Check sheet for the modelled part. Datum: model origin and axes. Units: mm. Face numbers are marked on the shaded views. A direction names the side the tool comes from. Give positions to 0.01 mm unless a question says otherwise; leave off trailing zeros. Write each loop counter-clockwise with the first axis right and the second up, starting at its lowest first coordinate (ties: lowest second). Pieces come first, ordered by that corner, then holes.
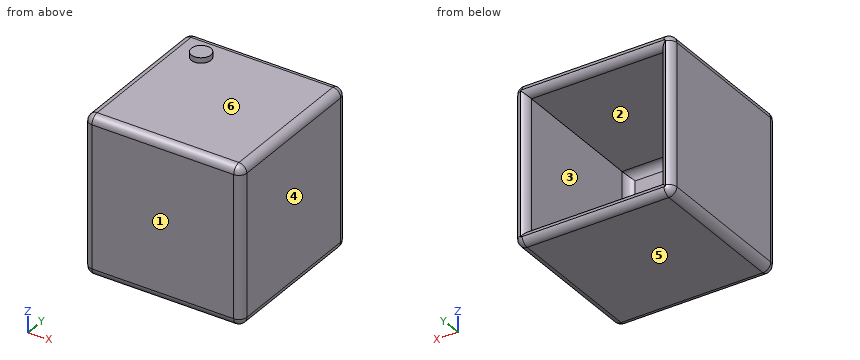
from build123d import *

# Parameters (mm, degrees)
F0_W         = 100
F0_H         = 100
F1_DEPTH     = 100
F2_R         = 5
F3_W         = 84.485553205
F3_H         = 83.5751444101
F4_DEPTH     = 96.9
F5_R         = 5
F6_T1_DEPTH  = 84.485553205
F6_T3_DEPTH  = 83.5751444101
F6_T9_DEPTH  = 96.985553205
F6_T13_DEPTH = 96.0751444101
F6_T20_DEPTH = 96.985553205
F6_T24_DEPTH = 96.0751444101
F6_T31_DEPTH = 96.0751444101
F6_T35_DEPTH = 96.985553205
F6_T42_DEPTH = 96.0751444101
F6_T46_DEPTH = 96.985553205
F7_R         = 6.1934205271
F8_DEPTH     = 3.4


# Not quite as in the source:
# - a fillet or chamfer that OpenCascade refuses, or shapes differently, is made with other operations: its cross-section is extruded or revolved along the edge and cut away or added


with BuildPart() as f1:
    # F0 (on Front) → F1 (new body)
    with BuildSketch(Plane.XZ):
        Rectangle(F0_W, F0_H)
    extrude(amount=F1_DEPTH)

    # F2
    f2_edges = [f1.edges().sort_by_distance(p)[0] for p in [
        (0, -100, 50),
        (-50, -100, 0),
        (0, -100, -50),
        (50, -100, 0),
        (50, -50, -50),
        (-50, -50, -50),
        (0, 0, -50),
        (50, -50, 50),
        (-50, -50, 50),
        (0, 0, 50),
        (50, 0, 0),
        (-50, 0, 0),
    ]]
    fillet(f2_edges, radius=F2_R)

    # F3 (on Front) → F4 (cut)
    with BuildSketch(Plane.XZ):
        Rectangle(F3_W, F3_H)
    extrude(amount=F4_DEPTH, mode=Mode.SUBTRACT)

    # F5
    f5_edges = [f1.edges().sort_by_distance(p)[0] for p in [
        (0, -96.9, -41.787572),
        (42.242777, -96.9, 0),
        (0, -96.9, 41.787572),
        (-42.242777, -96.9, 0),
    ]]
    fillet(f5_edges, radius=F5_R)

    # F6: fillet of radius 5 on 8 edges, made by hand

    # F6_s2 → F6_t1 (cut)
    with BuildSketch(Plane.YZ.offset(-42.2427766025)):
        with BuildLine():
            ThreePointArc((-5, -41.7875722051), (-1.4644660941, -43.2520382991), (0, -46.7875722051))
            Line((0, -46.7875722051), (0, -41.7875722051))
            Line((0, -41.7875722051), (-5, -41.7875722051))
        make_face()
        with BuildLine():
            ThreePointArc((0, 46.7875722051), (-1.4644660941, 43.2520382991), (-5, 41.7875722051))
            Line((-5, 41.7875722051), (0, 41.7875722051))
            Line((0, 41.7875722051), (0, 46.7875722051))
        make_face()
    extrude(amount=F6_T1_DEPTH, mode=Mode.SUBTRACT)

    # F6_s4 → F6_t3 (cut)
    with BuildSketch(Plane.XY.offset(-41.7875722051)):
        with BuildLine():
            ThreePointArc((47.2427766025, 0), (43.7072426966, -1.4644660941), (42.2427766025, -5))
            Line((42.2427766025, -5), (42.2427766025, 0))
            Line((42.2427766025, 0), (47.2427766025, 0))
        make_face()
        with BuildLine():
            ThreePointArc((-42.2427766025, -5), (-43.7072426966, -1.4644660941), (-47.2427766025, 0))
            Line((-47.2427766025, 0), (-42.2427766025, 0))
            Line((-42.2427766025, 0), (-42.2427766025, -5))
        make_face()
    extrude(amount=F6_T3_DEPTH, mode=Mode.SUBTRACT)


with BuildPart() as f6_tool7:
    # F6_s8 → F6_t9 (new body)
    with BuildSketch(Plane.YZ.offset(-54.7427766025)):
        with BuildLine():
            ThreePointArc((-5, -41.7875722051), (-1.4644660941, -43.2520382991), (0, -46.7875722051))
            Line((0, -46.7875722051), (0, -41.7875722051))
            Line((0, -41.7875722051), (-5, -41.7875722051))
        make_face()
    extrude(amount=F6_T9_DEPTH)

    split(bisect_by=Plane.YZ.offset(-42.2427766025), keep=Keep.BOTTOM)


with BuildPart() as f6_tool11:
    # F6_s12 → F6_t13 (new body)
    with BuildSketch(Plane.XY.offset(41.7875722051)):
        with BuildLine():
            ThreePointArc((-42.2427766025, -5), (-43.7072426966, -1.4644660941), (-47.2427766025, 0))
            Line((-47.2427766025, 0), (-42.2427766025, 0))
            Line((-42.2427766025, 0), (-42.2427766025, -5))
        make_face()
    extrude(amount=-F6_T13_DEPTH)

    split(bisect_by=Plane.XY.offset(-41.7875722051), keep=Keep.BOTTOM)


with BuildPart() as f6_tool7_1:
    add(f6_tool7.part)

    # F6_t15: intersect F6_tool11
    add(f6_tool11.part, mode=Mode.INTERSECT)


with BuildPart() as f1_1:
    add(f1.part)

    # F6_t5: cut F6_tool7
    add(f6_tool7_1.part, mode=Mode.SUBTRACT)


with BuildPart() as f6_tool18:
    # F6_s19 → F6_t20 (new body)
    with BuildSketch(Plane.YZ.offset(-42.2427766025)):
        with BuildLine():
            ThreePointArc((-5, -41.7875722051), (-1.4644660941, -43.2520382991), (0, -46.7875722051))
            Line((0, -46.7875722051), (0, -41.7875722051))
            Line((0, -41.7875722051), (-5, -41.7875722051))
        make_face()
    extrude(amount=F6_T20_DEPTH)

    split(bisect_by=Plane.YZ.offset(42.2427766025), keep=Keep.TOP)


with BuildPart() as f6_tool22:
    # F6_s23 → F6_t24 (new body)
    with BuildSketch(Plane.XY.offset(-54.2875722051)):
        with BuildLine():
            ThreePointArc((47.2427766025, 0), (43.7072426966, -1.4644660941), (42.2427766025, -5))
            Line((42.2427766025, -5), (42.2427766025, 0))
            Line((42.2427766025, 0), (47.2427766025, 0))
        make_face()
    extrude(amount=F6_T24_DEPTH)

    split(bisect_by=Plane.XY.offset(-41.7875722051), keep=Keep.BOTTOM)


with BuildPart() as f6_tool18_1:
    add(f6_tool18.part)

    # F6_t26: intersect F6_tool22
    add(f6_tool22.part, mode=Mode.INTERSECT)


with BuildPart() as f1_2:
    add(f1_1.part)

    # F6_t16: cut F6_tool18
    add(f6_tool18_1.part, mode=Mode.SUBTRACT)


with BuildPart() as f6_tool29:
    # F6_s30 → F6_t31 (new body)
    with BuildSketch(Plane.XY.offset(-41.7875722051)):
        with BuildLine():
            ThreePointArc((47.2427766025, 0), (43.7072426966, -1.4644660941), (42.2427766025, -5))
            Line((42.2427766025, -5), (42.2427766025, 0))
            Line((42.2427766025, 0), (47.2427766025, 0))
        make_face()
    extrude(amount=F6_T31_DEPTH)

    split(bisect_by=Plane.XY.offset(41.7875722051), keep=Keep.TOP)


with BuildPart() as f6_tool33:
    # F6_s34 → F6_t35 (new body)
    with BuildSketch(Plane.YZ.offset(54.7427766025)):
        with BuildLine():
            ThreePointArc((0, 46.7875722051), (-1.4644660941, 43.2520382991), (-5, 41.7875722051))
            Line((-5, 41.7875722051), (0, 41.7875722051))
            Line((0, 41.7875722051), (0, 46.7875722051))
        make_face()
    extrude(amount=-F6_T35_DEPTH)

    split(bisect_by=Plane.YZ.offset(42.2427766025), keep=Keep.TOP)


with BuildPart() as f6_tool29_1:
    add(f6_tool29.part)

    # F6_t37: intersect F6_tool33
    add(f6_tool33.part, mode=Mode.INTERSECT)


with BuildPart() as f1_3:
    add(f1_2.part)

    # F6_t27: cut F6_tool29
    add(f6_tool29_1.part, mode=Mode.SUBTRACT)


with BuildPart() as f6_tool40:
    # F6_s41 → F6_t42 (new body)
    with BuildSketch(Plane.XY.offset(54.2875722051)):
        with BuildLine():
            ThreePointArc((-42.2427766025, -5), (-43.7072426966, -1.4644660941), (-47.2427766025, 0))
            Line((-47.2427766025, 0), (-42.2427766025, 0))
            Line((-42.2427766025, 0), (-42.2427766025, -5))
        make_face()
    extrude(amount=-F6_T42_DEPTH)

    split(bisect_by=Plane.XY.offset(41.7875722051), keep=Keep.TOP)


with BuildPart() as f6_tool44:
    # F6_s45 → F6_t46 (new body)
    with BuildSketch(Plane.YZ.offset(42.2427766025)):
        with BuildLine():
            ThreePointArc((0, 46.7875722051), (-1.4644660941, 43.2520382991), (-5, 41.7875722051))
            Line((-5, 41.7875722051), (0, 41.7875722051))
            Line((0, 41.7875722051), (0, 46.7875722051))
        make_face()
    extrude(amount=-F6_T46_DEPTH)

    split(bisect_by=Plane.YZ.offset(-42.2427766025), keep=Keep.BOTTOM)


with BuildPart() as f6_tool40_1:
    add(f6_tool40.part)

    # F6_t48: intersect F6_tool44
    add(f6_tool44.part, mode=Mode.INTERSECT)


with BuildPart() as f1_4:
    add(f1_3.part)

    # F6_t38: cut F6_tool40
    add(f6_tool40_1.part, mode=Mode.SUBTRACT)

    # F7 (on face) → F8 (join)
    with BuildSketch(Plane.XY.offset(50)):
        with Locations((-29.7398809344, -18.3617770672)):
            Circle(F7_R)
    extrude(amount=F8_DEPTH)


solid = f1_4.part
1) Access from +Z, -Z, +X, -X, +Y, -Y to the whole of each face (thin tool, end or side, straight path). Record for the marked faces 1 and 2.
2) Sectioned sample at A-A on y = -38. Record the boundary of the cut face in (x, z), then the cut area to 3 significant figures.
3) Scan lines: L1, parallel to Z at x = -41, y = -60.5; L2, parallel to X at y = -50, z = -14.5; L3, parallel to Y at x = -12, z = 8.5. Record each from-to range of solid material in increasing order.
4) Sectioned sample at D-D on x = -34. Record the boundary of the cut face in (y, z), then the cut area to 3 significant figures.
5) Sectioned sample at B-B on z = 14. Record the boundary of the cut face in (x, y).
6) Sectioned sample at C-C on x = 10. Record the boundary of the cut face in (y, z).
7) Draft check along Z on the marked faces 3, 4, 5 and 6. Enter one of: +Z half, -Z half, draft (parallel to the pull), parting line (faces both ways), or undercut.
8) Gauge pin test, flat end, axial feed: pin 1 (1 mm diameter, centred on x = 22.5, y = -13, fed in from +Z). Record the tip position at first contact, or that the pin passes through.
Answers below:
1. face 1: +Z, -Z, +X, -X, -Y
1. face 2: +Y
2. outline: (-50, -45) arc R5 ccw to (-45, -50) - (45, -50) arc R5 ccw to (50, -45) - (50, 45) arc R5 ccw to (45, 50) - (-45, 50) arc R5 ccw to (-50, 45) - close; hole (-42.24, -41.79) - (42.24, -41.79) - (42.24, 41.79) - (-42.24, 41.79) - close
2. area: 2,920 mm2
3. L1: z = -50 to -41.79, 41.79 to 50
3. L2: x = -50 to -42.24, 42.24 to 50
3. L3: y = -100 to -96.9
4. outline: (-100, -45) arc R5 ccw to (-95, -50) - (-5, -50) arc R5 ccw to (-0.08, -45.89) arc R5 ccw to (-5, -41.79) - (-91.9, -41.79) arc R5 cw to (-96.9, -36.79) - (-96.9, 36.79) arc R5 cw to (-91.9, 41.79) - (-5, 41.79) arc R5 ccw to (-0.08, 45.89) arc R5 ccw to (-5, 50) - (-13.87, 50) - (-13.87, 53.4) - (-22.86, 53.4) - (-22.86, 50) - (-95, 50) arc R5 ccw to (-100, 45) - close
4. area: 1,910 mm2
5. outline: (-50, -95) arc R5 ccw to (-45, -100) - (45, -100) arc R5 ccw to (50, -95) - (50, -5) arc R5 ccw to (46.12, -0.13) arc R5 ccw to (42.24, -5) - (42.24, -91.9) arc R5 cw to (37.24, -96.9) - (-37.24, -96.9) arc R5 cw to (-42.24, -91.9) - (-42.24, -5) arc R5 ccw to (-46.12, -0.13) arc R5 ccw to (-50, -5) - close
6. outline: (-100, -45) arc R5 ccw to (-95, -50) - (-5, -50) arc R5 ccw to (-0.08, -45.89) arc R5 ccw to (-5, -41.79) - (-91.9, -41.79) arc R5 cw to (-96.9, -36.79) - (-96.9, 36.79) arc R5 cw to (-91.9, 41.79) - (-5, 41.79) arc R5 ccw to (-0.08, 45.89) arc R5 ccw to (-5, 50) - (-95, 50) arc R5 ccw to (-100, 45) - close
7. face 3: undercut
7. face 4: draft
7. face 5: -Z half
7. face 6: +Z half
8. pin 1: stops at z = 50
